The model under review builds one solid part; all positions refer to its coordinate system, in mm. A direction names the side the tool comes from. Give positions to 0.01 mm unless a question says otherwise; leave off trailing zeros. Order: outer loops, then holes, each group sorted by start corner. A loop starts at its lowest first (then second) coordinate and runs counter-clockwise, first axis right, second up. Notation, with made-up numbers: (-31, 75.5) - (-25, 75.5) arc R27 cw to (-25, 95.5) - close; hole circle Ø9 at (64.25, 75). An arc over 180 degrees is marked (long way). Use a Markdown table: item, result. Add a question column.
Autodesk Inventor part; units mm, degrees
ref_plane "Work Plane1" through (0, 0, 10) normal (0, 0, 1) x (1, 0, 0)
ref_plane "YZ Plane" through (0, 0, 0) normal (1, 0, 0) x (0, 1, 0)
ref_plane "XZ Plane" through (0, 0, 0) normal (0, 1, 0) x (-1, 0, 0)
sketch "Sketch1" plane through (0, 0, 0) normal (0, 0, 1) x (1, 0, 0)
  line L0 (0, 8) -> (0, -6)
  line L1 (-24.9804, 0) -> (33.3072, 0)
  line L2 (-20.817, 5) -> (20.817, 5)
  line L3 (20.817, 5) -> (20.817, -5)
  line L4 (20.817, -5) -> (-20.817, -5)
  line L5 (-20.817, -5) -> (-20.817, 5)
  dimension "d0" = 41.634
  dimension "d1" = 10
extrude "Extrusion1" add sketch "Sketch1" along normal blind 10
sketch "Sketch5" plane through (-20.817, -5, 0) normal (0, -1, 0) x (1, 0, 0)
  line L0 (41.634, 10) -> (0, 10)
  line L1 (18.817, 8) -> (22.817, 8)
  line L2 (22.817, 8) -> (22.817, 5)
  line L3 (22.817, 5) -> (18.817, 5)
  line L4 (18.817, 5) -> (18.817, 8)
  point P0 (20.817, 8)
  point P1 (20.817, 10)
  dimension "d20" = 4
  dimension "d21" = 3
  dimension "d22" = 2
extrude "Extrusion5" add sketch "Sketch5" along normal blind 1
ref_plane "Work Plane1" through (0, 0, 10) normal (0, 0, 1) x (1, 0, 0)
sketch "Sketch11" plane through (0, 0, 10) normal (0, 0, 1) x (1, 0, 0)
  line L0 (-17.217, -4.6) -> (-20.417, -4.6)
  line L1 (-20.417, -4.6) -> (-20.417, -0.2)
  line L2 (-20.417, -0.2) -> (-17.217, -0.2)
  line L3 (-17.217, -0.2) -> (-17.217, -4.6)
extrude "Extrusion11" cut sketch "Sketch11" against normal blind 7
pattern_linear "Rectangular Pattern3" count 10 spacing 4.182 along (1, 0, 0) count 2 spacing 4.8 along (0, 1, 0) of "Extrusion11"
properties part number "Power Supply Header 1"
Q1. Draft analysis for pull direction Y (two halves, no side actions). For faces 1 (the flat face through (0, 0, 10)), 2 (the flat face through (16.239, 2, 7)), state which applies: pulls with the +Y half, pulls with the -Y half, needs draft (parallel to the pull), parting line crosses it, or undercut.
Q2. We need section C-C (z = 2.5). Write out the cut boundary in (x, y), plus the area to 3 significant figures.
Q3. We need section B-B (z = 8.5). Count the separate pieces of the cut face and the enclosed holes in it, plus the area to 3 significant figures.
Q4. Machinability: for faces 3 (the flat face through (0, 0, 0)), 4 (the flat face through (-10, -0.2, 7)), which of the approach directions +Z, -Z, +X, -X, +Y, -Y give a long, thin tool a straight path to every point of the face, cutting with its end or side? Answer none if there is none.
Q5. Clearance check with flat-ended pins moving along their axes: P1, Ø1, axis at x = -2.5, y = -1.5, coming from the +Z side; P2, Ø1.1, axis at y = -5.5, z = 6.5, coming from the +X side; P3, Ø1.6, axis at x = -6, z = 8, coming from the -Y side. State where each tip first meets the part, or that it passes through.
Q6. We need section A-A (x = -1). Write out the cut boundary in (y, z), plus the area to 3 significant figures.
Q7. Wall thickness on probe 1 along Y at (x, z) = (6, 3.5); probe 2 along Y at (x, z) = (-17.5, 2.75); probe 3 along Z at (x, y) = (6, -1): over which ranges is each line inside the solid? List them lowest first.
Here are the results:
| question | item | result |
|---|---|---|
| 1 | face 1 | needs draft |
| 1 | face 2 | undercut |
| 2 | outline | (-20.82, -5) - (20.82, -5) - (20.82, 5) - (-20.82, 5) - close |
| 2 | area | 416 mm2 |
| 3 | separate pieces | 1 |
| 3 | enclosed holes | 20 |
| 3 | area | 135 mm2 |
| 4 | face 3 | -Z, +X, -X, +Y, -Y |
| 4 | face 4 | +Z |
| 5 | P1 | z = 3 |
| 5 | P2 | x = 20.82 |
| 5 | P3 | y = -5 |
| 6 | outline | (-6, 5) - (-5, 5) - (-5, 0) - (5, 0) - (5, 10) - (4.6, 10) - (4.6, 3) - (0.2, 3) - (0.2, 10) - (-0.2, 10) - (-0.2, 3) - (-4.6, 3) - (-4.6, 10) - (-5, 10) - (-5, 8) - (-6, 8) - close |
| 6 | area | 41.4 mm2 |
| 7 | probe 1 | -5 to -4.6, -0.2 to 0.2, 4.6 to 5 |
| 7 | probe 2 | -5 to 5 |
| 7 | probe 3 | 0 to 3 |
